from build123d import *

# Parameters (mm, degrees)
BOSS_EXTRUDE1_DEPTH = 2
SKETCH4_R           = 1.999996
CUT_EXTRUDE2_DEPTH  = 3


with BuildPart() as part:
    # Sketch2 → Boss-Extrude1 (new body)
    with BuildSketch(Plane.XY):
        with BuildLine():
            Line((369.86928226, 192.180584327), (358.0270208, 180.34))
            Line((358.0270208, 180.34), (268.1110208, 180.34))
            Line((268.1110208, 180.34), (255.978033197, 192.47289829))
            ThreePointArc((255.978033197, 192.47289829), (263.741388347, 198.123056954), (272.0624988, 202.913996))
            Line((272.0624988, 202.913996), (272.0624988, 193.261996))
            Line((272.0624988, 193.261996), (277.7630208, 185.928))
            Line((277.7630208, 185.928), (347.8670208, 185.928))
            Line((347.8670208, 185.928), (353.9630208, 194.056))
            Line((353.9630208, 194.056), (353.9630208, 202.64014406))
            ThreePointArc((353.9630208, 202.64014406), (362.193484504, 197.832115291), (369.86928226, 192.180584327))
        make_face()
    extrude(amount=BOSS_EXTRUDE1_DEPTH)

    # Sketch4 → Cut-Extrude2 (cut, through all)
    with BuildSketch(Plane(origin=(0, 0, 0), x_dir=(-1, 0, 0), z_dir=(0, 0, -1))):
        with Locations((-359.0430208, 194.564)):
            Circle(SKETCH4_R)
        with Locations((-359.0430208, 185.928)):
            Circle(SKETCH4_R)
        with Locations((-267.0950208, 185.928)):
            Circle(SKETCH4_R)
        with Locations((-267.0950208, 195.072)):
            Circle(SKETCH4_R)
    extrude(amount=-CUT_EXTRUDE2_DEPTH, mode=Mode.SUBTRACT)

    # Sketch5 → Loft4 section 0
    with BuildSketch(Plane.XY.offset(2)):
        Polygon((272.0624988, 193.261996), (272.0624988, 180.34), (353.9630208, 180.34), (353.9630208, 194.056), (347.8670208, 185.928), (277.7630208, 185.928), align=None)
    # Sketch6 → Loft4 section 1
    with BuildSketch(Plane.XY.offset(8)):
        Polygon((272.0624988, 202.913996), (272.0624988, 193.261996), (353.9630208, 194.056), (353.9630208, 202.64014406), (352.808404878, 202.184642252), (272.968388735, 202.184642252), align=None)
    loft()


solid = part.part
Verification items for the finished model (mm, model axes). A direction names the side the tool comes from. Round coordinates to 2 decimals unless told otherwise and drop trailing zeros. Use a Markdown table: item, result. Add a question column.
1. Thickness scan on probe 1 along Y at (x, z) = (341, 1); probe 2 along X at (y, z) = (190, 3); probe 3 along X at (y, z) = (194.5, 7.5). Record the ranges inside material, lowest first. Write a range as [from, to].
2. Gauge pin test, flat ends, axial feed: pin 1 (8 mm diameter, centred on x = 290.5, y = 192, fed in from -Z); pin 2 (12.5 mm diameter, centred on x = 363, y = 194.5, fed in from +Z); pin 3 (0.6 mm diameter, centred on y = 199, z = 0.5, fed in from -X). Record the tip position at first contact, or that the pin passes through.
3. Release check for a two-part mould opening along Y. For faces 4 (the face through (274.87, 189.65, 0.99)), 5 (the face through (266, 192, 2)), 6 (the face through (268.68, 184.71, 0.99)), 7 (the face through (262.13, 186.32, 0.99)) record: released by +Y, released by -Y, zero draft, split by the parting line, or undercut.
4. Access from +Z, -Z, +X, -X, +Y, -Y to the whole of each face (thin tool, end or side, straight path). Record for faces 1 (the face through (360, 192, 2)), 2 (the face through (313, 183, 0)), 3 (the face through (353.963, 198, 1)).
5. Section check A-A, the plane y = 200.5. Give the number of separate pieces and of enclosed holes in the cut face, plus the area to 3 significant figures.
Checks:
| question | item | result |
|---|---|---|
| 1 | probe 1 | y = [180.34, 185.93] |
| 1 | probe 2 | x = [272.06, 275.89], [349.74, 353.96] |
| 1 | probe 3 | x = [272.06, 353.96] |
| 2 | pin 1 | stops at z = 2.76 |
| 2 | pin 2 | stops at z = 2 |
| 2 | pin 3 | stops at x = 264.64 |
| 3 | face 4 | released by +Y |
| 3 | face 5 | zero draft |
| 3 | face 6 | undercut |
| 3 | face 7 | released by -Y |
| 4 | face 1 | +Z, +X, +Y, -Y |
| 4 | face 2 | -Z, +X, -X, +Y, -Y |
| 4 | face 3 | -Z, +Y |
| 5 | separate pieces | 3 |
| 5 | enclosed holes | 0 |
| 5 | area | 68.9 mm^2 |
